```python
from build123d import *

# Parameters (mm, degrees)
EXTRUDE_1_DEPTH       = 14
CUT_EXTRUDE_START     = 3
SKETCH_3_W            = 16
SKETCH_3_H            = 33.4
CUT_EXTRUDE_1_DEPTH   = 30.455434224
HOLE_WIZARD_7_0_7_1_D = 7


with BuildPart() as part:
    # 草图1 → 拉伸-薄壁1 (new, symmetric)
    with BuildSketch(Plane(origin=(0, 0, 0), x_dir=(0, 0, -1), z_dir=(1, 0, 0))):
        with BuildLine():
            Line((-16.7, 0), (-7.8, 0))
            ThreePointArc((-7.8, 0), (-4.759440841, 1.259440841), (-3.5, 4.3))
            Line((-3.5, 4.3), (-3.5, 12))
            ThreePointArc((-3.5, 12), (-2.621320344, 14.121320344), (-0.5, 15))
            Line((-0.5, 15), (0.5, 15))
            ThreePointArc((0.5, 15), (2.621320344, 14.121320344), (3.5, 12))
            Line((3.5, 12), (3.5, 4.3))
            ThreePointArc((3.5, 4.3), (4.759440841, 1.259440841), (7.8, 0))
            Line((7.8, 0), (16.7, 0))
            Line((16.7, 0), (16.7, 1.3))
            Line((16.7, 1.3), (7.8, 1.3))
            ThreePointArc((7.8, 1.3), (5.678679656, 2.178679656), (4.8, 4.3))
            Line((4.8, 4.3), (4.8, 12))
            ThreePointArc((4.8, 12), (3.540559159, 15.040559159), (0.5, 16.3))
            Line((0.5, 16.3), (-0.5, 16.3))
            ThreePointArc((-0.5, 16.3), (-3.540559159, 15.040559159), (-4.8, 12))
            Line((-4.8, 12), (-4.8, 4.3))
            ThreePointArc((-4.8, 4.3), (-5.678679656, 2.178679656), (-7.8, 1.3))
            Line((-7.8, 1.3), (-16.7, 1.3))
            Line((-16.7, 1.3), (-16.7, 0))
        make_face()
    extrude(amount=EXTRUDE_1_DEPTH, both=True)

    # 草图3 → 切除-拉伸1 (cut, through all)
    with BuildSketch(Plane(origin=(0, 1.3, 0), x_dir=(1, 0, 0), z_dir=(0, 1, 0)).offset(CUT_EXTRUDE_START)):
        with Locations((6, 0)):
            Rectangle(SKETCH_3_W, SKETCH_3_H)
    extrude(amount=-CUT_EXTRUDE_1_DEPTH, mode=Mode.SUBTRACT)

    # Ø7.0 (7) 直径孔1 (through all)
    with Locations(Plane.XY.offset(4.8)):
        with Locations((8, 9.3)):
            Hole(HOLE_WIZARD_7_0_7_1_D / 2)


solid = part.part
```
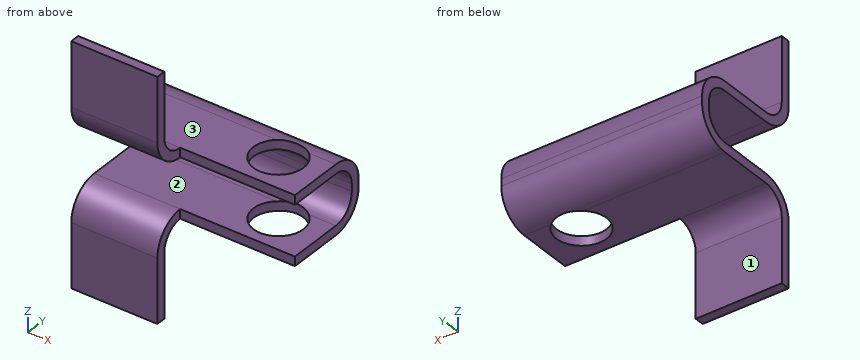
Model file for the job. Use its own axes, mm. Face numbers are marked on the shaded views. A direction names the side the tool comes from. Coordinates: 2 decimals unless noted, no trailing zeros. Order: outer loops, then holes, each group sorted by start corner. A loop starts at its lowest first (then second) coordinate and runs counter-clockwise, first axis right, second up. Notation, with made-up numbers: (-24.75, -0.5) - (-10.75, -0.5) arc R30 ccw to (-10.75, 21.5) - close; hole circle Ø5 at (15, 10.5). An arc over 180 degrees is marked (long way). Return JSON: item names as keys, results as strings. Group by question number.
1) Saw through at D-D, the plane x = 8.5. Write the cut outline in (y, z).
2) Saw through at B-B, the plane x = -9.5. Write the cut outline in (y, z).
3) Tool access for the marked faces 1, 2 and 3: list every direction of +Z, -Z, +X, -X, +Y, -Y with a clear straight run to the whole face (end or side of a thin tool).
4) Saw through at C-C, the plane y = 2.75. Write the cut outline in (x, z).
5) Flat gauge pins, fed straight in: P1, Ø6, axis at x = 6, y = 7, coming from the +Z side; P2, Ø2.5, axis at x = -9.5, z = 12, coming from the +Y side; P3, Ø2, axis at y = 1.5, z = -12.5, coming from the +X side; P4, Ø5.5, axis at x = 8, y = 9.3, coming from the -Z side. Where does each tip first touch, or does it go through?
6) Saw through at A-A, the plane y = 9.3. Write the cut outline in (x, z), plus the area to 3 significant figures.
7) Probe line 1 (Z direction, x = -9.5, y = 8.75); line 2 (X direction, y = 9.3, z = -3.95); line 3 (Y direction, x = -8.75, z = 11.5). List the from-to ranges inside material, lowest first. Write a range as from..to.
Values found:
{
 "1": {"outline": "(4.3, -4.8) - (5.84, -4.8) - (5.84, -3.5) - (4.3, -3.5) - close; (4.3, 3.5) - (5.84, 3.5) - (5.84, 4.8) - (4.3, 4.8) - close; (12.76, -4.73) arc R4.3 ccw to (16.3, -0.5) - (16.3, 0.5) arc R4.3 ccw to (12.76, 4.73) - (12.76, 3.4) arc R3 cw to (15, 0.5) - (15, -0.5) arc R3 cw to (12.76, -3.4) - close"},
 "2": {"outline": "(0, -16.7) - (1.3, -16.7) - (1.3, -7.8) arc R3 cw to (4.3, -4.8) - (12, -4.8) arc R4.3 ccw to (16.3, -0.5) - (16.3, 0.5) arc R4.3 ccw to (12, 4.8) - (4.3, 4.8) arc R3 cw to (1.3, 7.8) - (1.3, 16.7) - (0, 16.7) - (0, 7.8) arc R4.3 ccw to (4.3, 3.5) - (12, 3.5) arc R3 cw to (15, 0.5) - (15, -0.5) arc R3 cw to (12, -3.5) - (4.3, -3.5) arc R4.3 ccw to (0, -7.8) - close"},
 "3": {"face 1": "-Z, +X, -X, +Y", "face 2": "+X, -X, -Y", "face 3": "+Z, +X, -X, +Y"},
 "4": {"outline": "(-14, -5.23) - (-2, -5.23) - (-2, -3.79) - (-14, -3.79) - close; (-14, 3.79) - (-2, 3.79) - (-2, 5.23) - (-14, 5.23) - close"},
 "5": {"P1": "stops at z = 4.8", "P2": "stops at y = 1.3", "P3": "stops at x = -2", "P4": "passes through"},
 "6": {"outline": "(-14, -4.8) - (4.5, -4.8) - (4.5, -3.5) - (-14, -3.5) - close; (-14, 3.5) - (4.5, 3.5) - (4.5, 4.8) - (-14, 4.8) - close; (11.5, -4.8) - (14, -4.8) - (14, -3.5) - (11.5, -3.5) - close; (11.5, 3.5) - (14, 3.5) - (14, 4.8) - (11.5, 4.8) - close", "area": "54.6 mm²"},
 "7": {"line 1": "z = -4.8..-3.5, 3.5..4.8", "line 2": "x = -14..4.5, 11.5..14", "line 3": "y = 0..1.3"}
}
